Check sheet for the drawn part. Datum: minimum x, y, z corner. Units: mm. Coordinates: 2 decimals unless noted, no trailing zeros. Loops run counter-clockwise (first coordinate to the right, second up) from the corner with the lowest first, then second, coordinate; pieces in that order, holes last. Notation, with made-up numbers: (54, 47.25) -> (100, 47.25) arc R24 ccw to (100, 75.25) -> close; hole circle Ø2 at (88, 41.25). An arc over 180 degrees is marked (long way). Use CSV: the item, a comma, the result in double quotes. Start each with the question number.
1. Gauge pin test, flat end, axial feed: pin 1 (1 mm diameter, centred on x = 7, y = 15, fed in from -Z). Record the tip position at first contact, or that the pin passes through.
2. Thickness scan on L1, parallel to Z at x = 12, y = 34; L2, parallel to Y at x = 2.75, z = 42.5; L3, parallel to Y at x = 10, z = 18. Record the ranges inside material, lowest first.
3. Sectioned sample at A-A, the plane y = 47.5. Record the cut outline in (x, z), and give its area (3 significant figures).
4. Sectioned sample at B-B, the plane x = 10.5. Record the cut outline in (y, z) (1 decimal), and give its area (3 significant figures).
5. Sectioned sample at C-C, the plane z = 17.5. Record the cut outline in (x, y).
6. Sectioned sample at D-D, the plane y = 5. Record the cut outline in (x, z).
7. Release check for a two-part mould opening along Y. For the marked faces 1, 2, 3 and 4 record: pulls with the +Y half, pulls with the -Y half, needs draft (parallel to the pull), parting line crosses it, or undercut.
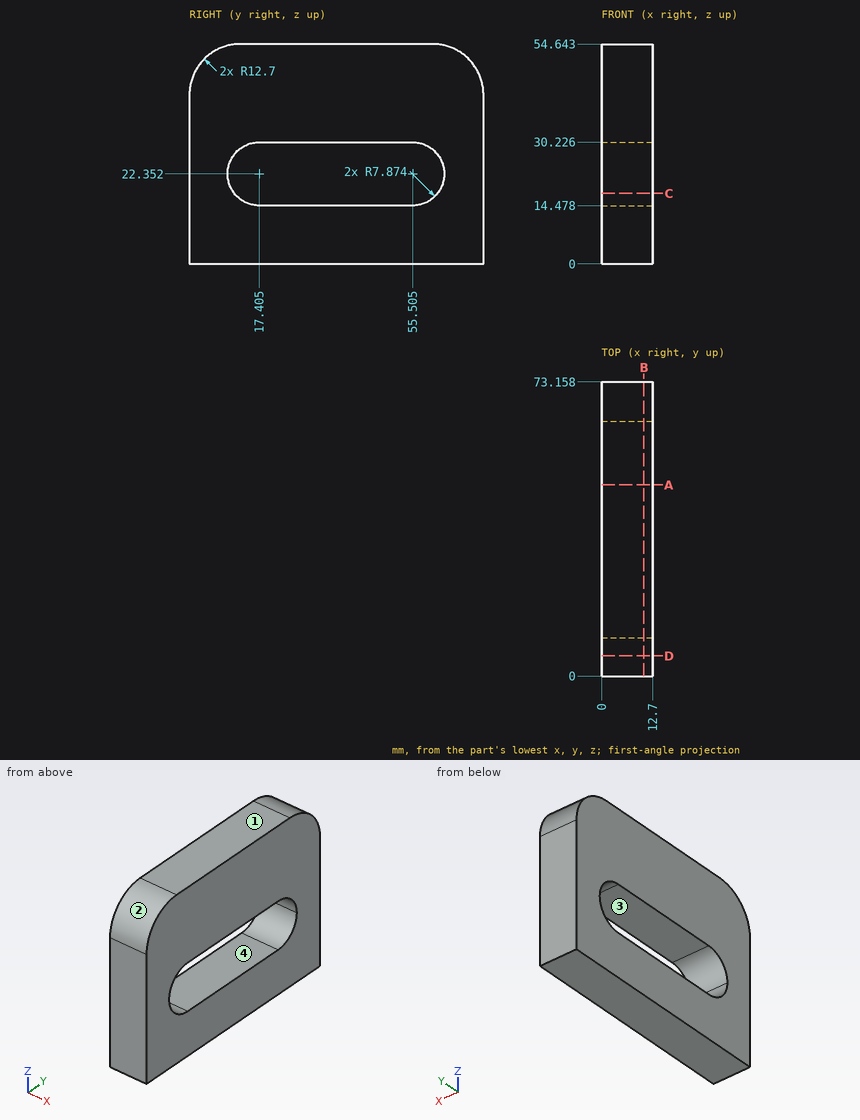
Completed:
1,pin 1,"z = 0"
2,L1,"0 to 14.48, 30.23 to 54.64"
2,L2,"0.01 to 73.15"
2,L3,"0 to 10.84, 62.07 to 73.16"
3,outline,"(0, 0) -> (12.7, 0) -> (12.7, 14.48) -> (0, 14.48) -> close; (0, 30.23) -> (12.7, 30.23) -> (12.7, 54.64) -> (0, 54.64) -> close"
3,area,"494 mm²"
4,outline,"(0, 0) -> (73.2, 0) -> (73.2, 41.9) arc R12.7 ccw to (60.5, 54.6) -> (12.7, 54.6) arc R12.7 ccw to (0, 41.9) -> close; hole (9.5, 22.4) arc R7.9 ccw to (17.4, 14.5) -> (55.5, 14.5) arc R7.9 ccw to (63.4, 22.4) arc R7.9 ccw to (55.5, 30.2) -> (17.4, 30.2) arc R7.9 ccw to start"
4,area,"3,130 mm²"
5,outline,"(0, 0) -> (12.7, 0) -> (12.7, 11.2) -> (0, 11.2) -> close; (0, 61.71) -> (12.7, 61.71) -> (12.7, 73.16) -> (0, 73.16) -> close"
6,outline,"(0, 0) -> (12.7, 0) -> (12.7, 52.04) -> (0, 52.04) -> close"
7,face 1,"needs draft"
7,face 2,"pulls with the -Y half"
7,face 3,"undercut"
7,face 4,"undercut"
